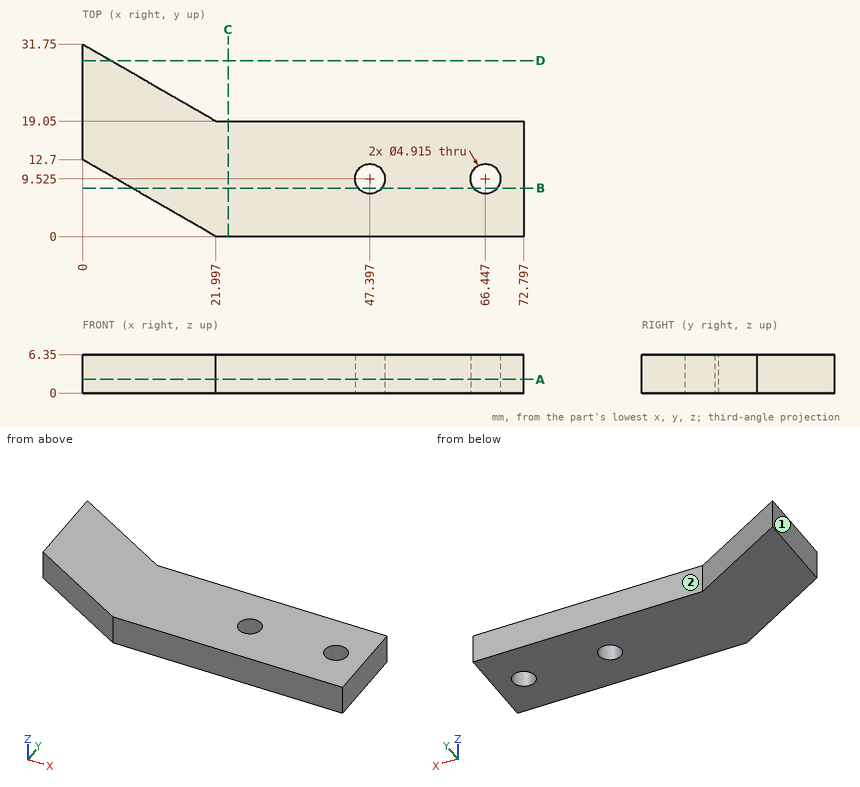
Geometry check sheet. Reference: drawing and pictorial views, mm from the part's lowest x, y, z. A direction names the side the tool comes from. Round coordinates to 2 decimals unless told otherwise and drop trailing zeros. Loops run counter-clockwise (first coordinate to the right, second up) from the corner with the lowest first, then second, coordinate; pieces in that order, holes last. Notation, with made-up numbers: (89, -16) - (148, -16) arc R28 ccw to (148, 9) - close; hole circle Ø7 at (-37.75, -10). An arc over 180 degrees is marked (long way). Answer in a Markdown table with one row per item. Add a question column.
Q1. Material ranges on line 1 (X direction, y = 11.5, z = 4.5) (1 decimal); line 2 (X direction, y = 9, z = 3.5); line 3 (Y direction, x = 51, z = 4.5), recorded low to high.
Q2. Section check C-C on x = 24. Enter the section's corners in (y, z), plus the area to 3 significant figures.
Q3. Tool access check on the marked faces 1 and 2. Record the directions out of +Z, -Z, +X, -X, +Y, -Y that give a thin tool (end or side, any length) a straight path to the whole face; none if there is none.
Q4. Section check A-A on z = 2.25. State how many separate pieces and enclosed holes the cut face has, plus the area to 3 significant figures.
Q5. Section check B-B on y = 8. Enter the section's corners in (x, z), plus the area to 3 significant figures.
Q6. Section check D-D on y = 29. Enter the section's corners in (x, z).
Q7. Gauge pin test, flat ends, axial feed: pin 1 (3 mm diameter, centred on x = 47.4, y = 9.52, fed in from -Z); pin 2 (1 mm diameter, centred on y = 15, z = 1.5, fed in from -X). Record the tip position at first contact, or that the pin passes through.
Found:
| question | item | result |
|---|---|---|
| 1 | line 1 | x = 2.1 to 45.9, 48.9 to 65, 67.9 to 72.8 |
| 1 | line 2 | x = 6.41 to 45, 49.8 to 64.05, 68.85 to 72.8 |
| 1 | line 3 | y = 0 to 19.05 |
| 2 | outline | (0, 0) - (19.05, 0) - (19.05, 6.35) - (0, 6.35) - close |
| 2 | area | 121 mm² |
| 3 | face 1 | +Z, -Z, -X, +Y, -Y |
| 3 | face 2 | +Z, -Z, +X, +Y |
| 4 | separate pieces | 1 |
| 4 | enclosed holes | 2 |
| 4 | area | 1,350 mm² |
| 5 | outline | (8.14, 0) - (45.47, 0) - (45.47, 6.35) - (8.14, 6.35) - close; (49.32, 0) - (64.52, 0) - (64.52, 6.35) - (49.32, 6.35) - close; (68.37, 0) - (72.8, 0) - (72.8, 6.35) - (68.37, 6.35) - close |
| 5 | area | 362 mm² |
| 6 | outline | (0, 0) - (4.76, 0) - (4.76, 6.35) - (0, 6.35) - close |
| 7 | pin 1 | passes through |
| 7 | pin 2 | stops at x = 0 |
